Design review of the part shown in the three views and the two pictorial views. Dimensions are in mm from the part's minimum x, y and z. A direction names the side the tool comes from. Coordinates: 2 decimals unless noted, no trailing zeros. Loops run counter-clockwise (first coordinate to the right, second up) from the corner with the lowest first, then second, coordinate; pieces in that order, holes last. Notation, with made-up numbers: (-27.75, 15) -> (-6.75, 15) arc R16 cw to (-6.75, 40) -> close; hole circle Ø3 at (9, 68.5). An arc over 180 degrees is marked (long way). One line per item, written item: value.
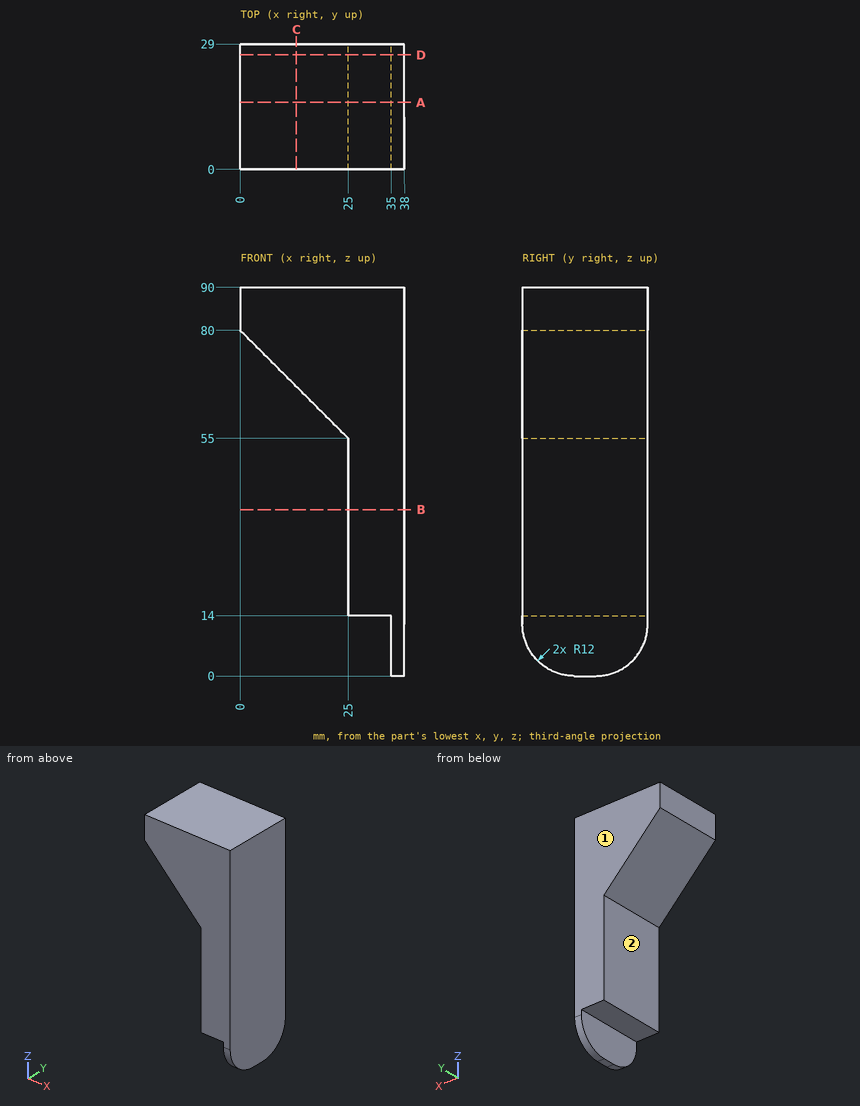
1. Take a section at C-C, the plane x = 13. Give the boundary of the cut face in (y, z), and give its area (3 significant figures).
Return value:
outline: (0, 67) -> (29, 67) -> (29, 90) -> (0, 90) -> close
area: 667 mm2
2. For the marked faces 1 and 2, list the 3-axis set-ups (+Z, -Z, +X, -X, +Y, -Y) from which the entire face can be reached by the end or side of a thin tool; tool diameter is ignored.
Return value:
face 1: +Z, -Z, +X, -X, +Y
face 2: -Z, -X, +Y, -Y
3. Insertion check: pin 1 Ø1 at (y, z) = (3.5, 56) entering from -X; pin 2 Ø7 at (y, z) = (14.5, 3.5) entering from -X; pin 3 Ø10 at (y, z) = (25.5, 43) entering from -X. Each pin has a flat end and moves straight along its axis. Give the tip position at first contact, or say it passes through.
Return value:
pin 1: stops at x = 23.5
pin 2: stops at x = 35
pin 3: stops at x = 25
4. To check wall thickness, follow probe 1 along X at (y, z) = (20.5, 10); probe 2 along Z at (x, y) = (26.5, 12.25); probe 3 along X at (y, z) = (3, 66). State the ranges of each line that lie inside material, in increasing order. Write a range as from..to.
Return value:
probe 1: x = 35..38
probe 2: z = 14..90
probe 3: x = 14..38
5. Take a section at B-B, the plane z = 38.5. Give the boundary of the cut face in (x, y).
Return value:
outline: (25, 0) -> (38, 0) -> (38, 29) -> (25, 29) -> close
6. Take a section at D-D, the plane y = 26.5. Give the boundary of the cut face in (x, z), and give its area (3 significant figures).
Return value:
outline: (0, 80) -> (25, 55) -> (25, 14) -> (35, 14) -> (35, 4.67) -> (38, 4.67) -> (38, 90) -> (0, 90) -> close
area: 1,580 mm2
7. Take a section at A-A, the plane y = 15.5. Give the boundary of the cut face in (x, z).
Return value:
outline: (0, 80) -> (25, 55) -> (25, 14) -> (35, 14) -> (35, 0) -> (38, 0) -> (38, 90) -> (0, 90) -> close
